Input: part model. Units: mm. Frame: model coordinates. A direction names the side the tool comes from. Coordinates: 2 decimals unless noted, no trailing zeros. Write each loop counter-clockwise with the first axis right and the second up, starting at its lowest first coordinate (ties: lowest second). Pieces come first, ordered by that corner, then holes. Notation, with made-up numbers: (59, 8.5) - (86, 8.5) arc R20 ccw to (86, 46.5) - close; hole circle Ø2 at (22.25, 20). An arc over 180 degrees is marked (long way). Put each result on its own line as item: value. Start each with the question number.
1. Cut plane A-A, the plane y = 7. Return loops of the section in (x, z), and give its area (3 significant figures).
2. Pull-direction query (Y, two-part tool) for faces 6 (the flat face through (-5.25, 30, 3)), 7 (the cylindrical face through (-43.954, 21.613, 2.465)), 8 (the flat face through (-9.6, 8, 3)), 9 (the flat face through (-14, 42.5, 2)); classes: released by +Y, released by -Y, zero draft, split by the parting line, or undercut.
3. Cut plane B-B, the plane x = -29. Return loops of the section in (y, z).
4. Cut plane C-C, the plane z = 1. Count the separate pieces of the cut face and the enclosed holes in it, and give its area (3 significant figures).
5. Line query: line 1 (Y direction, x = -36, z = 3.75); line 2 (Y direction, x = -29, z = 2.8); line 3 (X direction, y = 5.5, z = 1.7). Output: solid intervals per line, ascending.
6. Pin query (flat end, axial travel): pin 1 (2.5 mm diameter, centred on y = 2.5, z = 1.5, fed in from -X); pin 2 (2.5 mm diameter, centred on x = -11.5, z = 3, fed in from -Y); pin 3 (2.5 mm diameter, centred on x = -7.5, z = 3.5, fed in from +Y); pin 4 (1.3 mm diameter, centred on x = -5.5, z = 1.5, fed in from -Y). Return the tip coordinate at first contact, or that it passes through.
7. Access query for faces 1 (the flat face through (-11, 37.5, 2)), 2 (the flat face through (-16, 6, 2)), 3 (the flat face through (-16, 37, 2)), 4 (the flat face through (-11, 5, 3)), 5 (the flat face through (-10, 32.5, 3)). Directions: +Z, -Z, +X, -X, +Y, -Y. A direction counts if a zero-diameter tool reaches every point of the face in a straight line with its end or side. Return the directions, or none.
from build123d import *

# Parameters (mm, degrees)
BOSS_EXTRUDE1_DEPTH = 5
SKETCH2_R           = 5
SKETCH2_R_2         = 1
CUT_EXTRUDE1_DEPTH  = 10
SKETCH3_R           = 1
SKETCH3_R_2         = 1.440461169
BOSS_EXTRUDE2_DEPTH = 5
CUT_EXTRUDE2_DEPTH  = 10
SKETCH5_W           = 1
SKETCH5_H           = 5
CUT_EXTRUDE3_DEPTH  = 10


with BuildPart() as part:
    # Sketch1 → Boss-Extrude1 (new body)
    with BuildSketch(Plane.XY):
        with BuildLine():
            Line((-16, 31.40625), (-36, 31.40625))
            ThreePointArc((-36, 31.40625), (-46.15625, 21.25), (-36, 11.09375))
            Line((-36, 11.09375), (-16, 11.09375))
            Line((-16, 11.09375), (-16, 5))
            Line((-16, 5), (-16, 0))
            Line((-16, 0), (-11.25390625, 0))
            Line((-11.25390625, 0), (-11, 0))
            Line((-11, 0), (-11, 0.25390625))
            Line((-11, 0.25390625), (-11, 4.82421875))
            Line((-11, 4.82421875), (-11, 5))
            Line((-11, 5), (-10.74609375, 5))
            Line((-10.74609375, 5), (-8.20703125, 5))
            Line((-8.20703125, 5), (-5, 5))
            Line((-5, 5), (-5, 0))
            Line((-5, 0), (0, 0))
            Line((0, 0), (0, 42.5))
            Line((0, 42.5), (-5, 42.5))
            Line((-5, 42.5), (-5, 37.5))
            Line((-5, 37.5), (-8.20703125, 37.5))
            Line((-8.20703125, 37.5), (-10.74609375, 37.5))
            Line((-10.74609375, 37.5), (-11, 37.5))
            Line((-11, 37.5), (-11, 37.67578125))
            Line((-11, 37.67578125), (-11, 42.24609375))
            Line((-11, 42.24609375), (-11, 42.5))
            Line((-11, 42.5), (-11.25390625, 42.5))
            Line((-11.25390625, 42.5), (-16, 42.5))
            Line((-16, 42.5), (-16, 37.5))
            Line((-16, 37.5), (-16, 31.40625))
        make_face()
    extrude(amount=BOSS_EXTRUDE1_DEPTH)

    # Sketch2 → Cut-Extrude1 (cut)
    with BuildSketch(Plane(origin=(0, 0, 0), x_dir=(-1, 0, 0), z_dir=(0, 0, -1))):
        with Locations((36, 21.25)):
            Circle(SKETCH2_R)
        with Locations((43, 21.312454575)):
            Circle(SKETCH2_R_2)
        with Locations((36.062454575, 14.25)):
            Circle(SKETCH2_R_2)
        with Locations((29, 21.187545425)):
            Circle(SKETCH2_R_2)
        with Locations((35.937545425, 28.25)):
            Circle(SKETCH2_R_2)
    extrude(amount=-CUT_EXTRUDE1_DEPTH, mode=Mode.SUBTRACT)

    # Sketch3 → Boss-Extrude2 (add)
    with BuildSketch(Plane(origin=(0, 0, 0), x_dir=(-1, 0, 0), z_dir=(0, 0, -1))):
        with Locations((35.937545425, 28.25)):
            Circle(SKETCH3_R)
        with Locations((36.062454575, 14.25)):
            Circle(SKETCH3_R_2)
    extrude(amount=-BOSS_EXTRUDE2_DEPTH)

    # Sketch4 → Cut-Extrude2 (cut)
    with BuildSketch(Plane.XY.offset(5)):
        Polygon((-9.6, 5), (-6.4, 5), (-6.4, 10), (-5.25, 10), (-5.25, 14.5), (-10.75, 14.5), (-10.75, 10), (-9.6, 10), align=None)
        Polygon((-10.75, 32.5), (-10.75, 28), (-5.25, 28), (-5.25, 32.5), (-6.4, 32.5), (-6.4, 37.5), (-9.6, 37.5), (-9.6, 32.5), align=None)
    extrude(amount=-CUT_EXTRUDE2_DEPTH, mode=Mode.SUBTRACT)

    # Sketch5 → Cut-Extrude3 (cut)
    with BuildSketch(Plane.XY.offset(5)):
        with Locations((-4.5, 2.5)):
            Rectangle(SKETCH5_W, SKETCH5_H)
        with Locations((-11.5, 2.5)):
            Rectangle(SKETCH5_W, SKETCH5_H)
        with Locations((-11.5, 40)):
            Rectangle(SKETCH5_W, SKETCH5_H)
        with Locations((-4.5, 40)):
            Rectangle(SKETCH5_W, SKETCH5_H)
    extrude(amount=-CUT_EXTRUDE3_DEPTH, mode=Mode.SUBTRACT)


solid = part.part
Report:
1. outline: (-16, 0) - (-9.6, 0) - (-9.6, 5) - (-16, 5) - close; (-6.4, 0) - (0, 0) - (0, 5) - (-6.4, 5) - close
1. area: 64.0 mm^2
2. face 6: undercut
2. face 7: undercut
2. face 8: zero draft
2. face 9: released by +Y
3. outline: (11.09, 0) - (20.19, 0) - (20.19, 5) - (11.09, 5) - close; (22.19, 0) - (31.41, 0) - (31.41, 5) - (22.19, 5) - close
4. separate pieces: 1
4. enclosed holes: 3
4. area: 1,000 mm^2
5. line 1: y = 11.09 to 16.25, 26.25 to 31.41
5. line 2: y = 11.09 to 20.19, 22.19 to 31.41
5. line 3: x = -16 to -9.6, -6.4 to 0
6. pin 1: stops at x = -16
6. pin 2: stops at y = 0
6. pin 3: stops at y = 37.5
6. pin 4: stops at y = 5
7. face 1: +Z, -Z, +Y
7. face 2: +Z, -Z, -X, -Y
7. face 3: +Z, -Z, -X, +Y
7. face 4: +Z, -Z, -Y
7. face 5: +Z, -Z
